from build123d import *

# Parameters (mm, degrees)
F1_DEPTH      = 134.5
F1_DEPTH_BACK = 134.5
F2_R          = 2.5
F3_DEPTH      = 1
F3_TAPER      = -47.3248299171


with BuildPart() as f1:
    # F0 (on Right) → F1 (new body, two sides)
    with BuildSketch(Plane.YZ) as f1_sk:
        Polygon((-10, -5), (10, -5), (10, 5), (9, 5), (9, -4), (-9, -4), (-9, 5), (-10, 5), align=None)
    extrude(amount=F1_DEPTH)
    extrude(f1_sk.sketch, amount=-F1_DEPTH_BACK)

    # F2 (on face) → F3 (cut)
    with BuildSketch(Plane(origin=(0, 0, -5), x_dir=(1, 0, 0), z_dir=(0, 0, -1))):
        with Locations((-124, 0)):
            Circle(F2_R)
        with Locations((-95, 0)):
            Circle(F2_R)
    extrude(amount=-F3_DEPTH, taper=F3_TAPER, mode=Mode.SUBTRACT)


solid = f1.part
Input: part model. Units: mm. Frame: model coordinates. A direction names the side the tool comes from. Coordinates: 2 decimals unless noted, no trailing zeros. Order: outer loops, then holes, each group sorted by start corner. A loop starts at its lowest first (then second) coordinate and runs counter-clockwise, first axis right, second up.
1. Cut plane C-C, the plane y = 0. Count the separate pieces of the cut face and the enclosed holes in it, plus the area to 3 significant figures.
Checked values:
separate pieces: 3
enclosed holes: 0
area: 257 mm2
2. Cut plane B-B, the plane z = -0.5. Return loops of the section in (x, y), plus the area to 3 significant figures.
Checked values:
outline: (-134.5, -10) - (134.5, -10) - (134.5, -9) - (-134.5, -9) - close; (-134.5, 9) - (134.5, 9) - (134.5, 10) - (-134.5, 10) - close
area: 538 mm2
3. Ray query, line 1 along Y through (x, z) = (-120, 1.25); line 2 along Z through (x, y) = (-38, 7.75); line 3 along Z through (x, y) = (-98, 0). Return the intervals inside material, ascending.
Checked values:
line 1: y = -10 to -9, 9 to 10
line 2: z = -5 to -4
line 3: z = -5 to -4.54
4. Cut plane A-A, the plane x = -124. Return loops of the section in (y, z).
Checked values:
outline: (-10, -5) - (-2.5, -5) - (-3.58, -4) - (-9, -4) - (-9, 5) - (-10, 5) - close; (2.5, -5) - (10, -5) - (10, 5) - (9, 5) - (9, -4) - (3.58, -4) - close
5. Cut plane D-D, the plane x = -86.5. Return loops of the section in (y, z), plus the area to 3 significant figures.
Checked values:
outline: (-10, -5) - (10, -5) - (10, 5) - (9, 5) - (9, -4) - (-9, -4) - (-9, 5) - (-10, 5) - close
area: 38.0 mm2
6. Access query for faces 1 (the flat face through (-134.5, 0, -4.4)), 2 (the flat face through (2, -9, 0)). Directions: +Z, -Z, +X, -X, +Y, -Y. A direction counts if a zero-diameter tool reaches every point of the face in a straight line with its end or side. Return the directions, or none.
Checked values:
face 1: +Z, -Z, -X, +Y, -Y
face 2: +Z, +X, -X
